Part model, mm, in its own coordinate system. Face numbers are marked on the shaded views. A direction names the side the tool comes from. Coordinates: 2 decimals unless noted, no trailing zeros. Loops run counter-clockwise (first coordinate to the right, second up) from the corner with the lowest first, then second, coordinate; pieces in that order, holes last. Notation, with made-up numbers: (6, 81) -> (22, 81) arc R20 cw to (22, 112) -> close; hole circle Ø6 at (-13, -25). An arc over 180 degrees is marked (long way). Use one line per item in the form item = value. Start each with the question number.
(1) Pin check, flat tips, straight feed: P1, Ø2.5, axis at x = -37, y = 7, coming from the -Z side; P2, Ø2, axis at x = -38, z = 1.5, coming from the +Y side. Stop position of each tip, or through.
(2) Band-saw the part on D-D on z = 3.4. Give the cut face in (x, y), then the cut area to 3 significant figures.
(3) Drill centre lines: L1, parallel to Y at x = -4, z = 0.9; L2, parallel to Y at x = -23.5, z = 3.1; L3, parallel to Y at x = -46, z = 2.8. Where is each one in solid material? Low to high. Write a range as [from, to].
(4) 3-axis set-ups, long thin cutter, end or side, ignore diameter. For the marked faces 1 and 2: which of +Z, -Z, +X, -X, +Y, -Y reach the whole face in a straight line?
(5) Band-saw the part on A-A on y = 7. Give the cut face in (x, z), then the cut area to 3 significant figures.
(6) Band-saw the part on B-B on y = 42.5. Give the cut face in (x, z).
(7) Band-saw the part on C-C on x = -14. Give the cut face in (y, z), then the cut area to 3 significant figures.
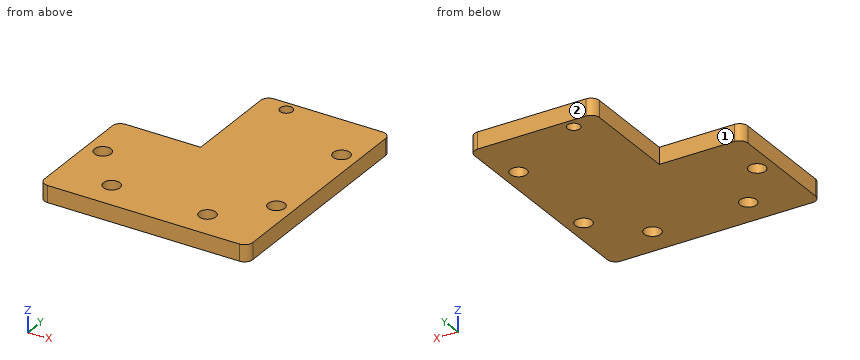
```python
from build123d import *

# Parameters (mm, degrees)
BOSS_EXTRUDE1_DEPTH = 4
FILLET1_R           = 2
SKETCH3_R           = 1.5
SKETCH3_R_2         = 2
CUT_EXTRUDE1_DEPTH  = 10


with BuildPart() as part:
    # Sketch1 → Boss-Extrude1 (new body)
    with BuildSketch(Plane.XY):
        Polygon((-30, 55), (0, 55), (0, 0), (-50, 0), (-50, 30), (-30, 30), align=None)
    extrude(amount=BOSS_EXTRUDE1_DEPTH)

    # Fillet1
    fillet1_edges = [part.edges().sort_by_distance(p)[0] for p in [
        (0, 0, 2),
        (-50, 0, 2),
        (-50, 30, 2),
        (-30, 55, 2),
        (0, 55, 2),
    ]]
    fillet(fillet1_edges, radius=FILLET1_R)

    # Sketch3 → Cut-Extrude1 (cut)
    with BuildSketch(Plane.XY.offset(4)):
        with Locations((-23.5, 52.5)):
            Circle(SKETCH3_R)
        with Locations((-46, 18)):
            Circle(SKETCH3_R_2)
        with Locations((-37, 7)):
            Circle(SKETCH3_R_2)
        with Locations((-14, 7)):
            Circle(SKETCH3_R_2)
        with Locations((-4, 17.5)):
            Circle(SKETCH3_R_2)
        with Locations((-4, 42.5)):
            Circle(SKETCH3_R_2)
    extrude(amount=-CUT_EXTRUDE1_DEPTH, mode=Mode.SUBTRACT)


solid = part.part
```
A:
q1.P1 = through
q1.P2 = 30
q2.outline = (-50, 2) arc R2 ccw to (-48, 0) -> (-2, 0) arc R2 ccw to (0, 2) -> (0, 53) arc R2 ccw to (-2, 55) -> (-28, 55) arc R2 ccw to (-30, 53) -> (-30, 30) -> (-48, 30) arc R2 ccw to (-50, 28) -> close; hole circle Ø4 at (-46, 18); hole circle Ø4 at (-37, 7); hole circle Ø3 at (-23.5, 52.5); hole circle Ø4 at (-14, 7); hole circle Ø4 at (-4, 17.5); hole circle Ø4 at (-4, 42.5)
q2.area = 2,180 mm²
q3.L1 = [0, 15.5], [19.5, 40.5], [44.5, 55]
q3.L2 = [0, 51], [54, 55]
q3.L3 = [0, 16], [20, 30]
q4.face_1 = +Z, -Z, -X, +Y
q4.face_2 = +Z, -Z, +X, -X, +Y
q5.outline = (-50, 0) -> (-39, 0) -> (-39, 4) -> (-50, 4) -> close; (-35, 0) -> (-16, 0) -> (-16, 4) -> (-35, 4) -> close; (-12, 0) -> (0, 0) -> (0, 4) -> (-12, 4) -> close
q5.area = 168 mm²
q6.outline = (-30, 0) -> (-6, 0) -> (-6, 4) -> (-30, 4) -> close; (-2, 0) -> (0, 0) -> (0, 4) -> (-2, 4) -> close
q7.outline = (0, 0) -> (5, 0) -> (5, 4) -> (0, 4) -> close; (9, 0) -> (55, 0) -> (55, 4) -> (9, 4) -> close
q7.area = 204 mm²
